Design review of the part shown in the three views and the two pictorial views. Dimensions are in mm from the part's minimum x, y and z. Coordinates: 2 decimals unless noted, no trailing zeros. Write item = value, one per line. Start each with the question number.
1) Draft analysis for pull direction Z (two halves, no side actions). For the marked faces 1, 2 and 3, state which applies: +Z half, -Z half, draft (parallel to the pull), parting line (faces both ways), or undercut.
2) Insertion check: pin 1 Ø10 at (x, z) = (33, 36.5) entering from -Y (3 decimals); pin 2 Ø18 at (x, z) = (28.5, 29) entering from -Y; pin 3 Ø3 at (x, y) = (30, 3) entering from -Z. Each pin has a flat end and moves straight along its axis. Give the tip position at first contact, or say it passes through.
3) Wall thickness on probe 1 along X at (y, z) = (0.05, 25.25); probe 2 along Y at (x, z) = (20, 16); probe 3 along Z at (x, y) = (6, 0.8): over which ranges is each line inside the solid? List them lowest first. Write a range as [from, to].
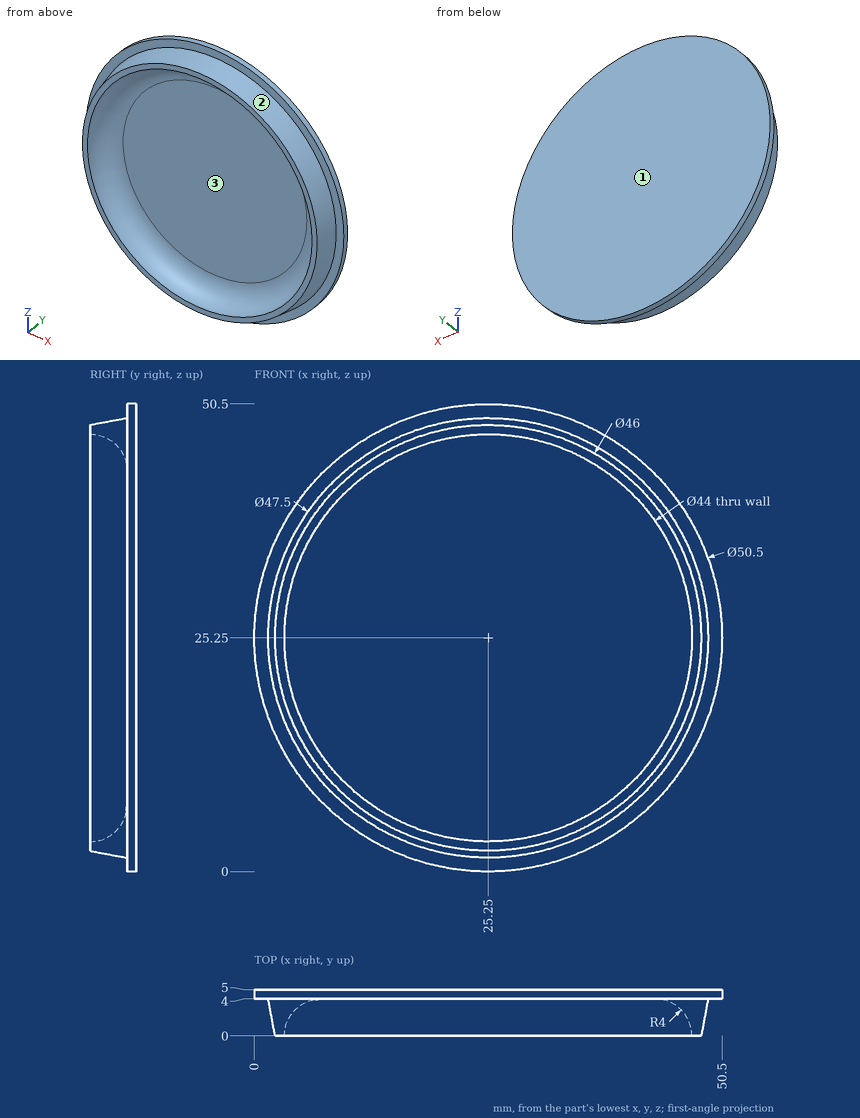
Answer sheet:
q1.face_1 = draft
q1.face_2 = parting line
q1.face_3 = undercut
q2.pin_1 = 3.945
q2.pin_2 = 4
q2.pin_3 = 0.26
q3.probe_1 = [2.24, 3.25], [47.25, 48.26]
q3.probe_2 = [4, 5]
q3.probe_3 = [12.39, 14.77], [35.73, 38.11]
